from build123d import *

# Parameters (mm, degrees)
SKETCH_1_W      = 10
SKETCH_1_H      = 45
SKETCH_1_R      = 2.653323097
SKETCH_1_R_2    = 2.5
EXTRUDE_1_DEPTH = 4


with BuildPart() as part:
    # 草圖1 → 填料-伸長1 (new body)
    with BuildSketch(Plane(origin=(0, 0, 0), x_dir=(1, 0, 0), z_dir=(0, 1, 0))):
        Rectangle(SKETCH_1_W, SKETCH_1_H)
        with Locations(Location((1.5, -2.055555556, 0), (0, 0, 270))):
            Circle(SKETCH_1_R, mode=Mode.SUBTRACT)
        with Locations(Location((1.5, -17.055555556, 0), (0, 0, 270))):
            Circle(SKETCH_1_R_2, mode=Mode.SUBTRACT)
        with BuildLine():
            Line((2.5, 18), (2.5, 7))
            ThreePointArc((2.5, 7), (0, 4.5), (-2.5, 7))
            Line((-2.5, 7), (-2.5, 18))
            ThreePointArc((-2.5, 18), (0, 20.5), (2.5, 18))
        make_face(mode=Mode.SUBTRACT)
    extrude(amount=EXTRUDE_1_DEPTH)


solid = part.part
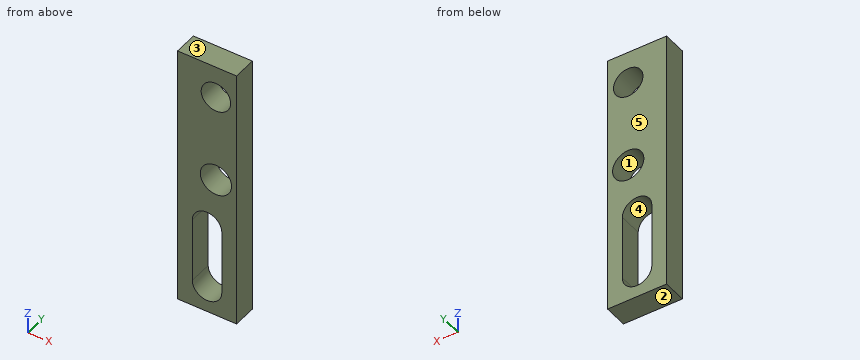
Geometry check sheet. Reference: the model listing, model coordinates, mm. Face numbers are marked on the shaded views. A direction names the side the tool comes from. Give positions to 0.01 mm unless a question says otherwise; leave off trailing zeros. Write each loop counter-clockwise with the first axis right and the second up, starting at its lowest first coordinate (ties: lowest second). Pieces come first, ordered by that corner, then holes.
1) Cross-section at B-B (x = 1.5). Record the boundary of the cut face in (y, z), plus the area to 3 significant figures.
Values follow:
outline: (0, -22.5) - (4, -22.5) - (4, -20) - (0, -20) - close; (0, -5) - (4, -5) - (4, -0.6) - (0, -0.6) - close; (0, 4.71) - (4, 4.71) - (4, 14.56) - (0, 14.56) - close; (0, 19.56) - (4, 19.56) - (4, 22.5) - (0, 22.5) - close
area: 78.8 mm2
2) Thickness scan on line 1 (Z direction, x = 3.5, y = 1.7); line 2 (X direction, y = 1.9, z = -12); line 3 (Z direction, x = 0.25, y = 2). Record the ranges inside material, lowest first.
Values follow:
line 1: z = -22.5 to 0.31, 3.8 to 15.56, 18.56 to 22.5
line 2: x = -5 to -2.5, 2.5 to 5
line 3: z = -22.5 to -20.49, -4.51 to -0.28, 4.4 to 14.89, 19.22 to 22.5
3) Release check for a two-part mould opening along Z. For the marked faces 1, 2 and 3 record: released by +Z, released by -Z, zero draft, split by the parting line, or undercut.
Values follow:
face 1: undercut
face 2: released by -Z
face 3: released by +Z
4) Cross-section at A-A (z = -8.5). Record the boundary of the cut face in (x, y), plus the area to 3 significant figures.
Values follow:
outline: (-5, 0) - (-2.5, 0) - (-2.5, 4) - (-5, 4) - close; (2.5, 0) - (5, 0) - (5, 4) - (2.5, 4) - close
area: 20.0 mm2
5) Cross-section at C-C (y = 1.4). Record the boundary of the cut face in (x, z), plus the area to 3 significant figures.
Values follow:
outline: (-5, -22.5) - (5, -22.5) - (5, 22.5) - (-5, 22.5) - close; hole (-2.5, -18) arc R2.5 ccw to (2.5, -18) - (2.5, -7) arc R2.5 ccw to (-2.5, -7) - close; hole circle Ø5.31 at (1.5, 2.06); hole circle Ø5 at (1.5, 17.06)
area: 334 mm2
6) Cross-section at D-D (x = 3.25). Record the boundary of the cut face in (y, z), plus the area to 3 significant figures.
Values follow:
outline: (0, -22.5) - (4, -22.5) - (4, 0.06) - (0, 0.06) - close; (0, 4.05) - (4, 4.05) - (4, 15.27) - (0, 15.27) - close; (0, 18.84) - (4, 18.84) - (4, 22.5) - (0, 22.5) - close
area: 150 mm2
7) Set-up check for the marked faces 4 and 5: record each of +Z, -Z, +X, -X, +Y, -Y from which the full face is reachable in a straight line by a thin tool's end or side.
Values follow:
face 4: +Y, -Y
face 5: +Z, -Z, +X, -X, +Y
